from build123d import *

# Parameters (mm, degrees)
SKETCH1_R           = 1.55
SKETCH1_R_2         = 1.4
BOSS_EXTRUDE1_DEPTH = 6
SKETCH2_R           = 39
SKETCH2_R_2         = 35.1
SKETCH2_R_3         = 33.1
CUT_EXTRUDE1_DEPTH  = 2


with BuildPart() as part:
    # Sketch1 → Boss-Extrude1 (new body)
    with BuildSketch(Plane.XY):
        with BuildLine():
            Line((-3.10553267, 45.170231176), (-4.343955751, 42.250868995))
            ThreePointArc((-4.343955751, 42.250868995), (-5.25243282, 41.063358876), (-6.621251333, 40.461821891))
            ThreePointArc((-6.621251333, 40.461821891), (-20.5, 35.507041555), (-31.730339975, 25.965082805))
            ThreePointArc((-31.730339975, 25.965082805), (-32.935695541, 25.080419692), (-34.418348006, 24.887410531))
            Line((-34.418348006, 24.887410531), (-37.565801358, 25.274585773))
            ThreePointArc((-37.565801358, 25.274585773), (-39.259871006, 24.987189905), (-40.518355186, 23.817281394))
            ThreePointArc((-40.518355186, 23.817281394), (-40.703193978, 23.5), (-40.88554833, 23.181284214))
            ThreePointArc((-40.88554833, 23.181284214), (-41.26947673, 21.506450688), (-40.671334028, 19.895645403))
            Line((-40.671334028, 19.895645403), (-38.762303757, 17.363458464))
            ThreePointArc((-38.762303757, 17.363458464), (-38.188128361, 15.982939184), (-38.351591308, 14.496739086))
            ThreePointArc((-38.351591308, 14.496739086), (-41, 0), (-38.351591308, -14.496739086))
            ThreePointArc((-38.351591308, -14.496739086), (-38.188128361, -15.982939184), (-38.762303757, -17.363458464))
            Line((-38.762303757, -17.363458464), (-40.671334028, -19.895645403))
            ThreePointArc((-40.671334028, -19.895645403), (-41.26947673, -21.506450688), (-40.88554833, -23.181284214))
            ThreePointArc((-40.88554833, -23.181284214), (-40.703193978, -23.5), (-40.518355186, -23.817281394))
            ThreePointArc((-40.518355186, -23.817281394), (-39.259871006, -24.987189905), (-37.565801358, -25.274585773))
            Line((-37.565801358, -25.274585773), (-34.418348006, -24.887410531))
            ThreePointArc((-34.418348006, -24.887410531), (-32.935695541, -25.080419692), (-31.730339975, -25.965082805))
            ThreePointArc((-31.730339975, -25.965082805), (-20.5, -35.507041555), (-6.621251333, -40.461821891))
            ThreePointArc((-6.621251333, -40.461821891), (-5.25243282, -41.063358876), (-4.343955751, -42.250868995))
            Line((-4.343955751, -42.250868995), (-3.10553267, -45.170231176))
            ThreePointArc((-3.10553267, -45.170231176), (-2.009605724, -46.493640593), (-0.367193143, -46.998565608))
            ThreePointArc((-0.367193143, -46.998565608), (0, -47), (0.367193143, -46.998565608))
            ThreePointArc((0.367193143, -46.998565608), (2.009605724, -46.493640593), (3.10553267, -45.170231176))
            Line((3.10553267, -45.170231176), (4.343955751, -42.250868995))
            ThreePointArc((4.343955751, -42.250868995), (5.25243282, -41.063358876), (6.621251333, -40.461821891))
            ThreePointArc((6.621251333, -40.461821891), (20.5, -35.507041555), (31.730339975, -25.965082805))
            ThreePointArc((31.730339975, -25.965082805), (32.935695541, -25.080419692), (34.418348006, -24.887410531))
            Line((34.418348006, -24.887410531), (37.565801358, -25.274585773))
            ThreePointArc((37.565801358, -25.274585773), (39.259871006, -24.987189905), (40.518355186, -23.817281394))
            ThreePointArc((40.518355186, -23.817281394), (40.703193978, -23.5), (40.88554833, -23.181284214))
            ThreePointArc((40.88554833, -23.181284214), (41.26947673, -21.506450688), (40.671334028, -19.895645403))
            Line((40.671334028, -19.895645403), (38.762303757, -17.363458464))
            ThreePointArc((38.762303757, -17.363458464), (38.188128361, -15.982939184), (38.351591308, -14.496739086))
            ThreePointArc((38.351591308, -14.496739086), (41, 0), (38.351591308, 14.496739086))
            ThreePointArc((38.351591308, 14.496739086), (38.188128361, 15.982939184), (38.762303757, 17.363458464))
            Line((38.762303757, 17.363458464), (40.671334028, 19.895645403))
            ThreePointArc((40.671334028, 19.895645403), (41.26947673, 21.506450688), (40.88554833, 23.181284214))
            ThreePointArc((40.88554833, 23.181284214), (40.703193978, 23.5), (40.518355186, 23.817281394))
            ThreePointArc((40.518355186, 23.817281394), (39.259871006, 24.987189905), (37.565801358, 25.274585773))
            Line((37.565801358, 25.274585773), (34.418348006, 24.887410531))
            ThreePointArc((34.418348006, 24.887410531), (32.935695541, 25.080419692), (31.730339975, 25.965082805))
            ThreePointArc((31.730339975, 25.965082805), (20.5, 35.507041555), (6.621251333, 40.461821891))
            ThreePointArc((6.621251333, 40.461821891), (5.25243282, 41.063358876), (4.343955751, 42.250868995))
            Line((4.343955751, 42.250868995), (3.10553267, 45.170231176))
            ThreePointArc((3.10553267, 45.170231176), (2.009605724, 46.493640593), (0.367193143, 46.998565608))
            ThreePointArc((0.367193143, 46.998565608), (0, 47), (-0.367193143, 46.998565608))
            ThreePointArc((-0.367193143, 46.998565608), (-2.009605724, 46.493640593), (-3.10553267, 45.170231176))
        make_face()
        with Locations((-0.063500562, 42.49999948)):
            Circle(SKETCH1_R, mode=Mode.SUBTRACT)
        with Locations((36.742579098, 21.24999948)):
            Circle(SKETCH1_R_2, mode=Mode.SUBTRACT)
        with Locations((36.742579098, -21.25000052)):
            Circle(SKETCH1_R_2, mode=Mode.SUBTRACT)
        with Locations((-0.063500562, -42.50000052)):
            Circle(SKETCH1_R_2, mode=Mode.SUBTRACT)
        with Locations((-36.869580223, -21.25000052)):
            Circle(SKETCH1_R_2, mode=Mode.SUBTRACT)
        with Locations((-36.869580223, 21.24999948)):
            Circle(SKETCH1_R_2, mode=Mode.SUBTRACT)
    extrude(amount=BOSS_EXTRUDE1_DEPTH)

    # Sketch2 → Cut-Extrude1 (cut)
    # profile 1 of 2: a face of its own
    with BuildSketch(Plane.XY.offset(6)):
        Circle(SKETCH2_R)
        Circle(SKETCH2_R_2, mode=Mode.SUBTRACT)
    # profile 2 of 2: a face of its own
    with BuildSketch(Plane.XY.offset(6)):
        Circle(SKETCH2_R_3)
    extrude(amount=-CUT_EXTRUDE1_DEPTH, mode=Mode.SUBTRACT)


solid = part.part
Read the model definition and answer for the solid it produces. Units are mm, in the model's axes. A direction names the side the tool comes from. Round coordinates to 2 decimals unless told otherwise and drop trailing zeros. Write each loop counter-clockwise with the first axis right and the second up, starting at its lowest first coordinate (ties: lowest second). Pieces come first, ordered by that corner, then holes.
1. Which of the six approach directions +Z, -Z, +X, -X, +Y, -Y give full straight-line access (tool end or side, diameter ignored) to faces 5 (the face through (-39.7, -18.61, 2.96)), 6 (the face through (-27.85, -21.36, 5.01)), 7 (the face through (39.73, -18.65, 2.96))?
2. Given pin 1 Ø3 at (y, z) = (-5, 3.5) entering from -X; pin 2 Ø1 at (y, z) = (27.5, 4) entering from -X; pin 3 Ø23.5 at (x, y) = (-16, 3) entering from +Z, each flat-ended and moving along its own axis, determine where each tip first touches the part or whether it passes through.
3. The part is cut by section B-B, the plane x = -19.5. Determine the outline of the cut face in (y, z) (3 decimals).
4. The part is cut by section D-D, the plane z = 2.6. State how many separate pieces and enclosed holes the cut face has, then the cut area to 3 significant figures.
5. The part is cut by section A-A, the plane y = 21.25. Determine the outline of the cut face in (x, z), then the cut area to 3 significant figures.
6. Straight lines are drawn through the part: L1, parallel to Y at x = 0, z = 2.65; L2, parallel to X at y = -21.25, z = 2.4; L3, parallel to Y at x = 28.5, z = 5.3. For each, find the intervals that lie inside material, in ascending order.
7. The part is cut by section C-C, the plane y = 0. Determine the outline of the cut face in (x, z), then the cut area to 3 significant figures.
8. Determine the mould class of faces 1 (the face through (-36.014, -25.084, 2.958)), 2 (the face through (3.733, 43.69, 2.958)), 3 (the face through (-5.27, -41.05, 2.96)), 4 (the face through (35.344, 21.312, 2.958)) for opening direction X: pulls with the +X half, pulls with the -X half, needs draft (parallel to the pull), parting line crosses it, or undercut.
Values:
1. face 5: +Z, -Z, -X
1. face 6: +Z
1. face 7: +Z, -Z, +X
2. pin 1: stops at x = -40.85
2. pin 2: stops at x = -30.85
2. pin 3: stops at z = 4
3. outline: (-36.066, 0) - (36.066, 0) - (36.066, 6) - (33.775, 6) - (33.775, 4) - (29.185, 4) - (29.185, 6) - (26.746, 6) - (26.746, 4) - (-26.746, 4) - (-26.746, 6) - (-29.185, 6) - (-29.185, 4) - (-33.775, 4) - (-33.775, 6) - (-36.066, 6) - close
4. separate pieces: 1
4. enclosed holes: 6
4. area: 5,500 mm2
5. outline: (-41.24, 0) - (-38.27, 0) - (-38.27, 6) - (-41.24, 6) - close; (-35.47, 0) - (35.34, 0) - (35.34, 6) - (32.7, 6) - (32.7, 4) - (27.94, 4) - (27.94, 6) - (25.38, 6) - (25.38, 4) - (-25.38, 4) - (-25.38, 6) - (-27.94, 6) - (-27.94, 4) - (-32.7, 4) - (-32.7, 6) - (-35.47, 6) - close; (38.14, 0) - (41.24, 0) - (41.24, 6) - (38.14, 6) - close
5. area: 341 mm2
6. L1: y = -47 to -43.9, -41.1 to 40.95, 44.05 to 47
6. L2: x = -41.24 to -38.27, -35.47 to 35.34, 38.14 to 41.24
6. L3: y = -29.47 to -26.62, -20.49 to -16.83, 16.83 to 20.49, 26.62 to 29.47
7. outline: (-41, 0) - (41, 0) - (41, 6) - (39, 6) - (39, 4) - (35.1, 4) - (35.1, 6) - (33.1, 6) - (33.1, 4) - (-33.1, 4) - (-33.1, 6) - (-35.1, 6) - (-35.1, 4) - (-39, 4) - (-39, 6) - (-41, 6) - close
7. area: 344 mm2
8. face 1: undercut
8. face 2: pulls with the +X half
8. face 3: pulls with the -X half
8. face 4: undercut
